Geometry: final body of the model. Coordinates: model frame, mm. A direction names the side the tool comes from. Give positions to 0.01 mm unless a question says otherwise; leave off trailing zeros. Loops run counter-clockwise (first coordinate to the right, second up) from the corner with the lowest first, then second, coordinate; pieces in that order, holes last. Notation, with made-up numbers: (9, 11.25) -> (29, 11.25) arc R18 ccw to (29, 22.25) -> close; hole circle Ø8 at (16.25, 10). An arc over 180 degrees is marked (long way). Answer in a Markdown table with one row per item. Add a question column.
from build123d import *

# Parameters (mm, degrees)
BOSS_EXTRUDE4_DEPTH = 5
BOSS_EXTRUDE5_DEPTH = 3.5
SKETCH2_R           = 11
CUT_EXTRUDE3_DEPTH  = 10
SKETCH2_4_R         = 11
SKETCH2_4_R_2       = 3.25
CUT_EXTRUDE4_DEPTH  = 25


with BuildPart() as part:
    # Sketch1 → Boss-Extrude4 (new, symmetric)
    with BuildSketch(Plane.XY):
        with BuildLine():
            ThreePointArc((-23.941610741, 7.197171327), (0, 25), (23.941610741, 7.197171327))
            Line((23.941610741, 7.197171327), (58.657369372, 21.57690938))
            ThreePointArc((58.657369372, 21.57690938), (42.267530451, 46.04026357), (16.495435726, 60.283916597))
            ThreePointArc((16.495435726, 60.283916597), (0, 62.5), (-16.495435726, 60.283916597))
            ThreePointArc((-16.495435726, 60.283916597), (-42.267530451, 46.04026357), (-58.657369372, 21.57690938))
            Line((-58.657369372, 21.57690938), (-23.941610741, 7.197171327))
        make_face()
        with BuildLine():
            ThreePointArc((16.495435726, 60.283916597), (42.267530451, 46.04026357), (58.657369372, 21.57690938))
            Line((58.657369372, 21.57690938), (70.213649137, 26.363677189))
            ThreePointArc((70.213649137, 26.363677189), (51.115143098, 54.883896965), (21.3105738, 71.908688239))
            Line((21.3105738, 71.908688239), (16.495435726, 60.283916597))
        make_face()
        with BuildLine():
            Line((-70.213649137, 26.363677189), (-58.657369372, 21.57690938))
            ThreePointArc((-58.657369372, 21.57690938), (-42.267530451, 46.04026357), (-16.495435726, 60.283916597))
            Line((-16.495435726, 60.283916597), (-21.3105738, 71.908688239))
            ThreePointArc((-21.3105738, 71.908688239), (-51.115143098, 54.883896965), (-70.213649137, 26.363677189))
        make_face()
        with BuildLine():
            ThreePointArc((16.495435726, -60.283916597), (42.267530451, -46.04026357), (58.657369372, -21.57690938))
            Line((58.657369372, -21.57690938), (23.941610741, -7.197171327))
            ThreePointArc((23.941610741, -7.197171327), (0, -25), (-23.941610741, -7.197171327))
            Line((-23.941610741, -7.197171327), (-58.657369372, -21.57690938))
            ThreePointArc((-58.657369372, -21.57690938), (-42.267530451, -46.04026357), (-16.495435726, -60.283916597))
            ThreePointArc((-16.495435726, -60.283916597), (0, -62.5), (16.495435726, -60.283916597))
        make_face()
        with BuildLine():
            ThreePointArc((-16.495435726, -60.283916597), (-42.267530451, -46.04026357), (-58.657369372, -21.57690938))
            Line((-58.657369372, -21.57690938), (-70.213649137, -26.363677189))
            ThreePointArc((-70.213649137, -26.363677189), (-51.115143098, -54.883896965), (-21.3105738, -71.908688239))
            Line((-21.3105738, -71.908688239), (-16.495435726, -60.283916597))
        make_face()
        with BuildLine():
            Line((70.213649137, -26.363677189), (58.657369372, -21.57690938))
            ThreePointArc((58.657369372, -21.57690938), (42.267530451, -46.04026357), (16.495435726, -60.283916597))
            Line((16.495435726, -60.283916597), (21.3105738, -71.908688239))
            ThreePointArc((21.3105738, -71.908688239), (51.115143098, -54.883896965), (70.213649137, -26.363677189))
        make_face()
    extrude(amount=BOSS_EXTRUDE4_DEPTH, both=True)

    # Sketch1_3 → Boss-Extrude5 (add, symmetric)
    with BuildSketch(Plane.XY):
        with BuildLine():
            Line((58.657369372, 21.57690938), (23.941610741, 7.197171327))
            ThreePointArc((23.941610741, 7.197171327), (0, 25), (-23.941610741, 7.197171327))
            Line((-23.941610741, 7.197171327), (-58.657369372, 21.57690938))
            ThreePointArc((-58.657369372, 21.57690938), (-62.5, 0), (-58.657369372, -21.57690938))
            Line((-58.657369372, -21.57690938), (-23.941610741, -7.197171327))
            ThreePointArc((-23.941610741, -7.197171327), (0, -25), (23.941610741, -7.197171327))
            Line((23.941610741, -7.197171327), (58.657369372, -21.57690938))
            ThreePointArc((58.657369372, -21.57690938), (61.53184373, -10.958202733), (62.5, 0))
            ThreePointArc((62.5, 0), (61.53184373, 10.958202733), (58.657369372, 21.57690938))
        make_face()
    extrude(amount=BOSS_EXTRUDE5_DEPTH, both=True)

    # Sketch2 → Cut-Extrude3 (cut)
    with BuildSketch(Plane.XY.offset(3.5)):
        Circle(SKETCH2_R)
    extrude(amount=-CUT_EXTRUDE3_DEPTH, mode=Mode.SUBTRACT)

    # Sketch2_4 → Cut-Extrude4 (cut)
    with BuildSketch(Plane.XY.offset(3.5)):
        Circle(SKETCH2_4_R)
        with Locations((48, 0)):
            Circle(SKETCH2_4_R_2)
        with Locations((41.569219382, -24)):
            Circle(SKETCH2_4_R_2)
        with Locations((24, -41.569219382)):
            Circle(SKETCH2_4_R_2)
        with Locations((0, -48)):
            Circle(SKETCH2_4_R_2)
        with Locations((-24, -41.569219382)):
            Circle(SKETCH2_4_R_2)
        with Locations((-41.569219382, -24)):
            Circle(SKETCH2_4_R_2)
        with Locations((-48, 0)):
            Circle(SKETCH2_4_R_2)
        with Locations((-41.569219382, 24)):
            Circle(SKETCH2_4_R_2)
        with Locations((-24, 41.569219382)):
            Circle(SKETCH2_4_R_2)
        with Locations((0, 48)):
            Circle(SKETCH2_4_R_2)
        with Locations((24, 41.569219382)):
            Circle(SKETCH2_4_R_2)
        with Locations((41.569219382, 24)):
            Circle(SKETCH2_4_R_2)
    extrude(amount=-CUT_EXTRUDE4_DEPTH, mode=Mode.SUBTRACT)


solid = part.part
(1) Cut plane D-D on y = 57. Return the cut outline in (x, z), then the cut area to 3 significant figures.
(2) Pin query (flat end, axial travel): pin 1 Ø3 at (x, y) = (-0.5, -48) entering from -Z; pin 2 Ø1.5 at (x, z) = (14.5, 0.5) entering from -Y; pin 3 Ø1 at (y, z) = (-48.5, 1.5) entering from -X. Return the tip coordinate at first contact, or that it passes through.
(3) Material intervals for line 1 along Y through (x, z) = (24, -0.5); line 2 along Y through (x, z) = (-44, -4.5); line 3 along X through (y, z) = (-25.5, 0.25), sorted ascending. Write a range as from..to.
(4) Cut plane A-A on x = -48. Return the cut outline in (y, z), then the cut area to 3 significant figures.
(5) Draft query along Y for faces 4 (the cylindrical face through (-0.2, -62.5, 0.1)), 5 (the cylindrical face through (-50.76, 55.21, -0.07)), 6 (the flat face through (24, 42, 3.5)). Return one class per face: +Y half, -Y half, draft (parallel to the pull), parting line (faces both ways), or undercut.
(6) Cut plane C-C on x = 0. Return the cut outline in (y, z).
(7) Reachability of faces 1 (the cylindrical face through (0, -25, 4)), 2 (the flat face through (18.937, 66.178, -0.07)), 3 (the cylindrical face through (44.571, -25.245, -0.691)) from +Z, -Z, +X, -X, +Y, -Y: full face, straight path, thin tool, end or side. Return the list, or none.
(8) Cut plane B-B on z = 1.75. State how many separate pieces and enclosed holes the cut face has, then the cut area to 3 significant figures.
Answer list:
| question | item | result |
|---|---|---|
| 1 | outline | (-48.74, -5) -> (48.74, -5) -> (48.74, 5) -> (-48.74, 5) -> close |
| 1 | area | 975 mm² |
| 2 | pin 1 | stops at z = 3.5 |
| 2 | pin 2 | stops at y = -60.97 |
| 2 | pin 3 | stops at x = -57.63 |
| 3 | line 1 | y = -71.06..-44.82, -38.32..38.32, 44.82..71.06 |
| 3 | line 2 | y = -60.74..-26.16, -21.84..-15.51, 15.51..21.84, 26.16..60.74 |
| 3 | line 3 | x = -68.13..-44.45, -38.69..38.69, 44.45..68.13 |
| 4 | outline | (-57.63, -5) -> (-17.16, -5) -> (-17.16, -3.5) -> (-3.25, -3.5) -> (-3.25, 3.5) -> (-17.16, 3.5) -> (-17.16, 5) -> (-57.63, 5) -> close; (3.25, -3.5) -> (17.16, -3.5) -> (17.16, -5) -> (57.63, -5) -> (57.63, 5) -> (17.16, 5) -> (17.16, 3.5) -> (3.25, 3.5) -> close |
| 4 | area | 1,000 mm² |
| 5 | face 4 | -Y half |
| 5 | face 5 | +Y half |
| 5 | face 6 | undercut |
| 6 | outline | (-62.5, -5) -> (-51.25, -5) -> (-51.25, 3.5) -> (-44.75, 3.5) -> (-44.75, -5) -> (-25, -5) -> (-25, -3.5) -> (-11, -3.5) -> (-11, 3.5) -> (-25, 3.5) -> (-25, 5) -> (-62.5, 5) -> close; (11, -3.5) -> (25, -3.5) -> (25, -5) -> (44.75, -5) -> (44.75, 3.5) -> (51.25, 3.5) -> (51.25, -5) -> (62.5, -5) -> (62.5, 5) -> (25, 5) -> (25, 3.5) -> (11, 3.5) -> close |
| 7 | face 1 | +Z |
| 7 | face 2 | +Z, -Z, +Y |
| 7 | face 3 | -Z |
| 8 | separate pieces | 1 |
| 8 | enclosed holes | 13 |
| 8 | area | 14,700 mm² |
